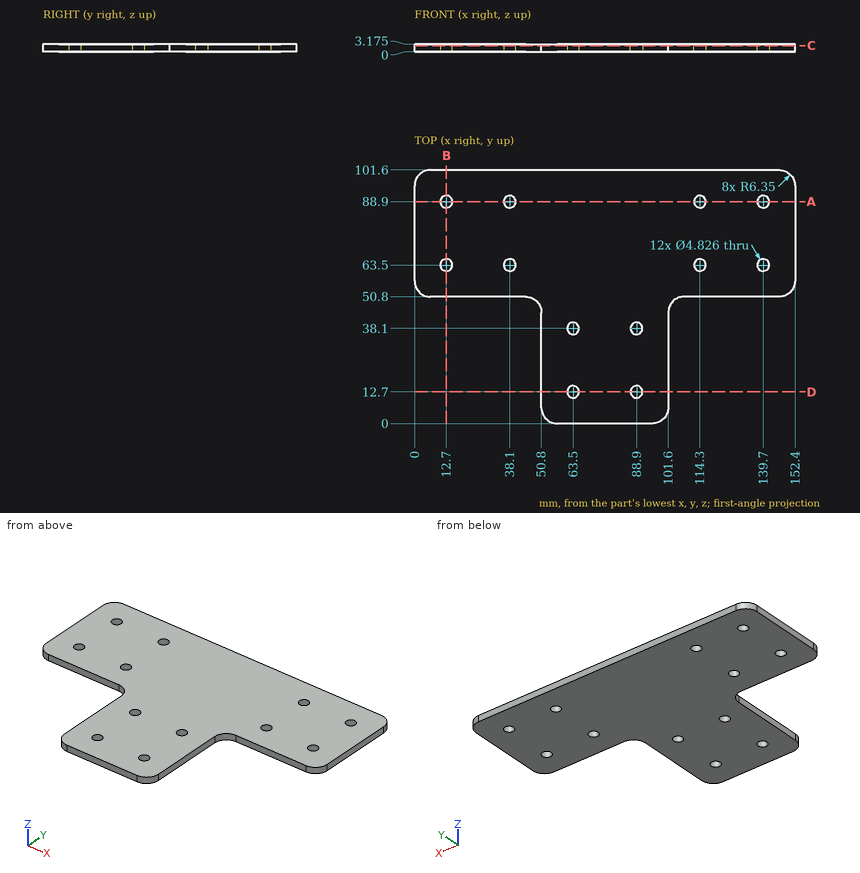
The figure shows three views and two pictorial views of one solid part (mm, origin at its lowest corner). Answer the questions. Round coordinates to 2 decimals unless told otherwise and drop trailing zeros. Write each loop counter-clockwise with the first axis right and the second up, starting at its lowest first coordinate (ties: lowest second). Pieces come first, ordered by that corner, then holes. Notation, with made-up numbers: (43, 32.5) - (68, 32.5) arc R12 cw to (68, 47.5) - close; hole circle Ø5 at (87.25, 44). An arc over 180 degrees is marked (long way). Answer in a Markdown table with one row per item. Add a question column.
1. Given pin 1 (5.5 mm diameter, centred on x = 88.9, y = 38.1, fed in from -Z); pin 2 (1.6 mm diameter, centred on y = 32, z = 1.5, fed in from +X); pin 3 (1 mm diameter, centred on x = 19, z = 1, fed in from -Y), each flat-ended and moving along its own axis, determine where each tip first touches the part or whether it passes through.
2. A cutting plane is placed at A-A, the plane y = 88.9. Determine the outline of the cut face in (x, z) (3 decimals), and give its area (3 significant figures).
3. A cutting plane is placed at C-C, the plane z = 2.5. Count the separate pieces of the cut face and the enclosed holes in it, and give its area (3 significant figures).
4. Find the intervals of material crossed by line 1 along Y through (x, z) = (38, 2.2); line 2 along Y through (x, z) = (63.5, 1.4); line 3 along X through (y, z) = (89, 0.85), in increasing order. Write a range as from..to.
5. A cutting plane is placed at B-B, the plane x = 12.7. Determine the outline of the cut face in (y, z) (3 decimals), and give its area (3 significant figures).
Worked out:
| question | item | result |
|---|---|---|
| 1 | pin 1 | z = 0 |
| 1 | pin 2 | x = 101.6 |
| 1 | pin 3 | y = 50.8 |
| 2 | outline | (0, 0) - (10.287, 0) - (10.287, 3.175) - (0, 3.175) - close; (15.113, 0) - (35.687, 0) - (35.687, 3.175) - (15.113, 3.175) - close; (40.513, 0) - (111.887, 0) - (111.887, 3.175) - (40.513, 3.175) - close; (116.713, 0) - (137.287, 0) - (137.287, 3.175) - (116.713, 3.175) - close; (142.113, 0) - (152.4, 0) - (152.4, 3.175) - (142.113, 3.175) - close |
| 2 | area | 423 mm^2 |
| 3 | separate pieces | 1 |
| 3 | enclosed holes | 12 |
| 3 | area | 10,100 mm^2 |
| 4 | line 1 | 50.8..61.09, 65.91..86.49, 91.31..101.6 |
| 4 | line 2 | 0..10.29, 15.11..35.69, 40.51..101.6 |
| 4 | line 3 | 0..10.29, 15.11..35.69, 40.51..111.89, 116.71..137.29, 142.11..152.4 |
| 5 | outline | (50.8, 0) - (61.087, 0) - (61.087, 3.175) - (50.8, 3.175) - close; (65.913, 0) - (86.487, 0) - (86.487, 3.175) - (65.913, 3.175) - close; (91.313, 0) - (101.6, 0) - (101.6, 3.175) - (91.313, 3.175) - close |
| 5 | area | 131 mm^2 |
